from build123d import *

# Parameters (mm, degrees)
EXTRUDE_1_DEPTH     = 3
SKETCH_8_R          = 12.5
EXTRUDE_2_DEPTH     = 3
SKETCH_2_R          = 3.5
CUT_EXTRUDE_1_DEPTH = 159.522080481
SKETCH_5_R          = 1.5
CUT_EXTRUDE_2_DEPTH = 159.522080481
FILLET_3_R          = 20
SKETCH_9_R          = 2
CUT_EXTRUDE_3_DEPTH = 159.522080481


with BuildPart() as part:
    # 草图1 → 凸台-拉伸1 (new body)
    with BuildSketch(Plane(origin=(0, 0, 0), x_dir=(1, 0, 0), z_dir=(0, 1, 0))):
        with BuildLine():
            Line((0, 8), (150, 8))
            ThreePointArc((150, 8), (158, 0), (150, -8))
            Line((150, -8), (0, -8))
            ThreePointArc((0, -8), (-8, 0), (0, 8))
        make_face()
    extrude(amount=EXTRUDE_1_DEPTH)

    # 草图8 → 凸台-拉伸2 (add)
    with BuildSketch(Plane(origin=(0, 3, 0), x_dir=(1, 0, 0), z_dir=(0, 1, 0))):
        with Locations((80, 0)):
            Circle(SKETCH_8_R)
    extrude(amount=-EXTRUDE_2_DEPTH)

    # 草图2 → 切除-拉伸1 (cut, through all)
    with BuildSketch(Plane(origin=(0, 3, 0), x_dir=(1, 0, 0), z_dir=(0, 1, 0))):
        with Locations(Location((80, 0, 0), (0, 0, 270))):
            Circle(SKETCH_2_R)
        with BuildLine():
            Line((84.456249475, 6.857459024), (85.516909647, 7.918119195))
            ThreePointArc((85.516909647, 7.918119195), (87.918119195, 7.918119195), (87.918119195, 5.516909647))
            Line((87.918119195, 5.516909647), (86.857459024, 4.456249475))
            ThreePointArc((86.857459024, 4.456249475), (84.456249475, 4.456249475), (84.456249475, 6.857459024))
        make_face()
        with BuildLine():
            Line((84.456249475, -6.857459024), (85.516909647, -7.918119195))
            ThreePointArc((85.516909647, -7.918119195), (87.918119195, -7.918119195), (87.918119195, -5.516909647))
            Line((87.918119195, -5.516909647), (86.857459024, -4.456249475))
            ThreePointArc((86.857459024, -4.456249475), (84.456249475, -4.456249475), (84.456249475, -6.857459024))
        make_face()
        with BuildLine():
            Line((73.142540976, -4.456249475), (72.081880805, -5.516909647))
            ThreePointArc((72.081880805, -5.516909647), (72.081880805, -7.918119195), (74.483090353, -7.918119195))
            Line((74.483090353, -7.918119195), (75.543750525, -6.857459024))
            ThreePointArc((75.543750525, -6.857459024), (75.543750525, -4.456249475), (73.142540976, -4.456249475))
        make_face()
        with BuildLine():
            Line((75.543750525, 6.857459024), (74.483090353, 7.918119195))
            ThreePointArc((74.483090353, 7.918119195), (72.081880805, 7.918119195), (72.081880805, 5.516909647))
            Line((72.081880805, 5.516909647), (73.142540976, 4.456249475))
            ThreePointArc((73.142540976, 4.456249475), (75.543750525, 4.456249475), (75.543750525, 6.857459024))
        make_face()
    extrude(amount=-CUT_EXTRUDE_1_DEPTH, mode=Mode.SUBTRACT)

    # 草图5 → 切除-拉伸2 (cut, through all)
    with BuildSketch(Plane(origin=(0, 3, 0), x_dir=(1, 0, 0), z_dir=(0, 1, 0))):
        with Locations(Location((10, 0, 0), (0, 0, 270))):
            Circle(SKETCH_5_R)
        with Locations(Location((0, 5, 0), (0, 0, 270))):
            Circle(SKETCH_5_R)
        with Locations(Location((0, -5, 0), (0, 0, 270))):
            Circle(SKETCH_5_R)
    extrude(amount=-CUT_EXTRUDE_2_DEPTH, mode=Mode.SUBTRACT)

    # 圆角3
    fillet_3_edges = [part.edges().sort_by_distance(p)[0] for p in [
        (70.395313644, 1.5, 8),
        (70.395313644, 1.5, -8),
        (89.604686356, 1.5, 8),
        (89.604686356, 1.5, -8),
    ]]
    fillet(fillet_3_edges, radius=FILLET_3_R)

    # 草图9 → 切除-拉伸3 (cut, through all)
    with BuildSketch(Plane(origin=(0, 3, 0), x_dir=(1, 0, 0), z_dir=(0, 1, 0))):
        with Locations(Location((150, 0, 0), (0, 0, 270))):
            Circle(SKETCH_9_R)
    extrude(amount=-CUT_EXTRUDE_3_DEPTH, mode=Mode.SUBTRACT)


solid = part.part
The listing builds one solid part. Answer for the finished solid, in the listing's coordinates (mm). A direction names the side the tool comes from. Coordinates: 2 decimals unless noted, no trailing zeros. Loops run counter-clockwise (first coordinate to the right, second up) from the corner with the lowest first, then second, coordinate; pieces in that order, holes last. Notation, with made-up numbers: (84, 58) -> (117, 58) arc R9 cw to (117, 64) -> close; hole circle Ø10 at (-33, 70). An arc over 180 degrees is marked (long way). Write item = value, one per line. Start each with the question number.
1) A cutting plane is placed at B-B (y = 0.65). Count the separate pieces of the cut face and the enclosed holes in it, then the cut area to 3 significant figures.
2) A cutting plane is placed at A-A (x = 10). Give the vertices of the cut face in (y, z), then the cut area to 3 significant figures.
3) A cutting plane is placed at D-D (x = 139). Give the vertices of the cut face in (y, z), then the cut area to 3 significant figures.
4) A cutting plane is placed at C-C (z = 0). Give the vertices of the cut face in (x, y), then the cut area to 3 significant figures.
5) The mould has two halves that part along Z. Classify faces 4 (the face through (31, 1, -8)), 5 (the face through (158, 1, 0)), 6 (the face through (8.536, 1.521, -0.325)), 7 (the face through (91.166, 1.521, 8.724)): released by +Z, released by -Z, zero draft, split by the parting line, or undercut.
6) Straight lines are drawn through the part: line 1 (X direction, y = 1.75, z = 0); line 2 (Z direction, x = -1, y = 2.8); line 3 (X direction, y = 1.1, z = -5) (3 decimals). For each, find the intervals that lie inside material, in ascending order. Write a range as from..to.
7) A tool of negligible diameter and unlimited length cuts with its end or side. For faces 1 (the face through (76.583, 1.521, -0.759)), 2 (the face through (124, 1, 8)), 3 (the face through (32, 1, 8)), from which of +Z, -Z, +X, -X, +Y, -Y can it reach the whole face along a straight path? Write none if from no direction.
8) Given pin 1 Ø1.8 at (x, z) = (10, 0) entering from -Y; pin 2 Ø1.5 at (x, y) = (19.5, 1) entering from -Z; pin 3 Ø0.9 at (x, y) = (37, 1.5) entering from +Z, each flat-ended and moving along its own axis, determine where each tip first touches the part or whether it passes through.
Responses:
q1.separate_pieces = 1
q1.enclosed_holes = 9
q1.area = 2,610 mm²
q2.outline = (0, -8) -> (3, -8) -> (3, -1.5) -> (0, -1.5) -> close; (0, 1.5) -> (3, 1.5) -> (3, 8) -> (0, 8) -> close
q2.area = 39.0 mm²
q3.outline = (0, -8) -> (3, -8) -> (3, 8) -> (0, 8) -> close
q3.area = 48.0 mm²
q4.outline = (-8, 0) -> (8.5, 0) -> (8.5, 3) -> (-8, 3) -> close; (11.5, 0) -> (76.5, 0) -> (76.5, 3) -> (11.5, 3) -> close; (83.5, 0) -> (148, 0) -> (148, 3) -> (83.5, 3) -> close; (152, 0) -> (158, 0) -> (158, 3) -> (152, 3) -> close
q4.area = 456 mm²
q5.face_4 = released by -Z
q5.face_5 = split by the parting line
q5.face_6 = undercut
q5.face_7 = released by +Z
q6.line_1 = -8..8.5, 11.5..76.5, 83.5..148, 152..158
q6.line_2 = -7.94..-6.12, -3.88..3.88, 6.12..7.94
q6.line_3 = -6.245..-1.5, 1.5..72.599, 75.909..84.091, 87.401..156.245
q7.face_1 = +Y, -Y
q7.face_2 = +Z, +X, +Y, -Y
q7.face_3 = +Z, -X, +Y, -Y
q8.pin_1 = through
q8.pin_2 = -8
q8.pin_3 = 8
